Autodesk Inventor part; units mm, degrees
ref_plane "YZ Plane" through (0, 0, 0) normal (1, 0, 0) x (0, 1, 0)
ref_plane "XZ Plane" through (0, 0, 0) normal (0, 1, 0) x (-1, 0, 0)
ref_plane "XY Plane" through (0, 0, 0) normal (0, 0, 1) x (1, 0, 0)
sketch "Sketch1" plane through (0, 0, 0) normal (0, 1, 0) x (-1, 0, 0)
  arc A0 (0, -5) -> (4.4, -2.3749) centre (0, 0) ccw
  line L0 (0, 0) -> (0, 29.6022) construction
  line L1 (10, 9.2633) -> (10, 13.6302)
  line L2 (2.254, 28) -> (-1.8447, 28)
  line L3 (9.4, 6.8883) -> (4.4, -2.3749)
  arc A1 (9.4, 6.8883) -> (10, 9.2633) centre (5, 9.2633) ccw
  arc A2 (-4.4, -2.3749) -> (0, -5) centre (0, 0) ccw
  line L4 (-10, 9.2633) -> (-10, 23)
  line L5 (-5, 28) -> (-1.8447, 28)
  line L6 (-9.4, 6.8883) -> (-4.4, -2.3749)
  arc A3 (-10, 9.2633) -> (-9.4, 6.8883) centre (-5, 9.2633) ccw
  arc A4 (-5, 28) -> (-10, 23) centre (-5, 23) ccw
  arc A5 (4.825, 18) -> (6.95, 15.875) centre (6.95, 18) ccw
  line L7 (4.825, 18) -> (4.825, 28)
  line L8 (4.825, 28) -> (2.254, 28)
  line L9 (10, 13.6302) -> (10, 15.875)
  line L10 (10, 15.875) -> (6.95, 15.875)
  circle A6 centre (0, 0) radius 5
  point P0 (10, 28)
  point P1 (10, 8)
  point P2 (-10, 28)
  dimension "d0" = 10
  dimension "d3" = 10
  dimension "d4" = 28
  dimension "d26" = 8
  dimension "d27" = 5
  dimension "d48" = 5
  dimension "d51" = 3.05
  dimension "d52" = 10
  dimension "d53" = 4.25
extrude "Extrusion1" add sketch "Sketch1" along normal blind 2
sketch "Sketch3" plane through (0, 2, 0) normal (0, 1, 0) x (1, 0, 0)
  line L0 (0, 0) -> (0, -24.7147) construction
  line L1 (-4.825, -28) -> (5, -28)
  arc A0 (9.25, -8) -> (4.75, -8) centre (7, -8) ccw
  circle A1 centre (-7, -13.5) radius 2.25
  line L2 (7, -8) -> (7, -11) construction
  line L3 (9.25, -8) -> (9.25, -11)
  line L4 (4.75, -11) -> (4.75, -8)
  arc A2 (9.25, -8) -> (4.75, -8) centre (7, -8) ccw
  arc A3 (4.75, -11) -> (9.25, -11) centre (7, -11) ccw
  arc A4 (-6.5467, -11.2961) -> (5.1678, -6.694) centre (-4.2232, 0) ccw
  line L5 (7.3955, -13.215) -> (-6.6045, -15.715)
  point P0 (-4, -28)
  point P1 (-2.254, -28)
  point P2 (7, -9.5)
  dimension "d28" = 20
  dimension "d29" = 7
  dimension "d46" = 7
  dimension "d47" = 14.5
  dimension "d96" = 4.5
  dimension "d97" = 4.5
  dimension "d136" = 3
fillet "Fillet1" radius 2 2 edges at (-10, 1, 15.875) (-4.825, 1, 28)
sketch "Sketch4" plane through (0, 0, 0) normal (0, -1, 0) x (1, 0, 0)
  point P0 (0, 0)
  point P1 (0, 25)
  dimension "d37" = 25
hole "Hole4" at (0, 0, 25) direction (0, 1, 0) diameter 3 end through all
sketch "Sketch5" plane through (0, 0, 0) normal (0, -1, 0) x (1, 0, 0)
  circle A0 centre (0, 25) radius 1.5
  circle A1 centre (0, 25) radius 1.5
  arc A2 (-2.825, 28) -> (-4.825, 26) centre (-2.825, 26) ccw
  line L0 (-4.825, 26) -> (-4.825, 18)
  arc A3 (-6.95, 15.875) -> (-4.825, 18) centre (-6.95, 18) ccw
  line L1 (-6.95, 15.875) -> (-8, 15.875)
  arc A4 (-8, 15.875) -> (-10, 13.875) centre (-8, 13.875) ccw
  line L2 (-10, 13.875) -> (-10, 9.2633)
  arc A5 (-10, 9.2633) -> (-9.4, 6.8883) centre (-5, 9.2633) ccw
  line L3 (-9.4, 6.8883) -> (-4.4, -2.3749)
  arc A6 (-4.4, -2.3749) -> (4.4, -2.3749) centre (0, 0) ccw
  line L4 (4.4, -2.3749) -> (9.4, 6.8883)
  arc A7 (9.4, 6.8883) -> (10, 9.2633) centre (5, 9.2633) ccw
  line L5 (10, 9.2633) -> (10, 23)
  arc A8 (10, 23) -> (5, 28) centre (5, 23) ccw
  line L6 (5, 28) -> (-2.825, 28)
  circle A9 centre (0, 25) radius 9.8995 construction
  line L7 (0, 25) -> (17.632, 25) construction
  line L8 (0, 25) -> (13.9609, 10.961) construction
  arc A10 (4.6888, 20.285) -> (10, 16.7785) centre (6.9804, 17.9805) ccw
  arc A11 (4.6888, 20.285) -> (5.9826, 27.9025) centre (0, 25) ccw
  dimension "d55" = 19.799
  dimension "d56" = 45.16
  dimension "d57" = 6.5
extrude "Extrusion2" cut sketch "Sketch5" against normal through all contours A8 L5 A10 A11
fillet "Fillet2" radius 3 1 edges at (5.9826, 1, 27.9025)
fillet "Fillet3" radius 2 1 edges at (10, 1, 16.7785)
extrude "Extrusion5" add sketch "Sketch3" against normal blind 6.75
sketch "Sketch14" plane through (0, 0, 0) normal (0, -1, 0) x (1, 0, 0)
  circle A0 centre (0, 0) radius 5
  dimension "d123" = 10
extrude "Extrusion6" add sketch "Sketch14" along normal blind 1
sketch "Sketch15" plane through (0, -1, 0) normal (0, -1, 0) x (1, 0, 0)
  circle A0 centre (0, 0) radius 4.75
  dimension "d126" = 9.5
extrude "Extrusion7" add sketch "Sketch15" along normal blind 2.1
sketch "Sketch16" plane through (0, 2, 0) normal (0, 1, 0) x (1, 0, 0)
  point P0 (0, 0)
  point P1 (0, 0)
hole "Hole11" at (0, 2, 0) direction (0, -1, 0) diameter 3 end through all
sketch "Sketch17" plane through (0, -4.75, 0) normal (0, -1, 0) x (1, 0, 0)
  arc A0 (-6.6045, 15.715) -> (-6.5467, 11.2961) centre (-7, 13.5) ccw
  arc A1 (5.1678, 6.694) -> (-6.5467, 11.2961) centre (-4.2232, 0) ccw
  arc A2 (5.1678, 6.694) -> (9.25, 8) centre (7, 8) ccw
  line L0 (9.25, 8) -> (9.25, 11)
  arc A3 (9.25, 11) -> (7.3955, 13.215) centre (7, 11) ccw
  line L1 (7.3955, 13.215) -> (-6.6045, 15.715)
  line L2 (7, 8) -> (7, 11) construction
  point P0 (0, 0)
  point P1 (7, 9.5)
hole "mounting" at (7, -4.75, 9.5) at (-7, -4.75, 13.5) direction (0, 1, 0) diameter 2 depth 5.5
properties part number "phalanx_2_housing_R"
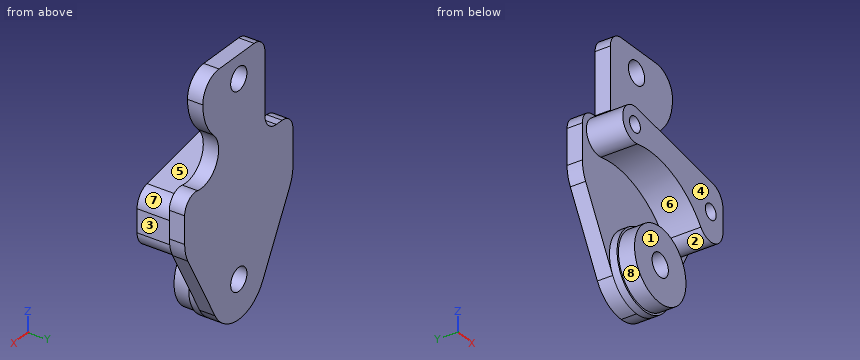
The model under review builds one solid part; all positions refer to its coordinate system, in mm. Face numbers are marked on the shaded views. A direction names the side the tool comes from. Give positions to 0.01 mm unless a question says otherwise; leave off trailing zeros. Order: outer loops, then holes, each group sorted by start corner. A loop starts at its lowest first (then second) coordinate and runs counter-clockwise, first axis right, second up. Notation, with made-up numbers: (-14, 32) - (32, 32) arc R22 ccw to (32, 70) - close; hole circle Ø4 at (73.5, 5). An arc over 180 degrees is marked (long way). Use CSV: the item, a comma, the result in double quotes. Start each with the question number.
Q1. The part is to be moulded in two halves that separate along X. For the marked faces 6, 7 and 8, say which applies: +X half, -X half, draft (parallel to the pull), parting line (faces both ways), or undercut.
Q2. We need section B-B, the plane x = 2.75. Write out the cut boundary in (y, z), and give its area (3 significant figures).
Q3. Tool access review of the marked faces 1, 2, 3, 4 and 5: name each direction out of +Z, -Z, +X, -X, +Y, -Y from which nothing blocks a thin tool from reaching the whole face with its end or side.
Q4. We need section C-C, the plane z = 2. Write out the cut boundary in (x, y).
Q5. We need section D-D, the plane x = 8.75. Write out the cut boundary in (y, z), and give its area (3 significant figures).
Q6. Clearance check with flat-ended pins moving along their axes: pin 1 Ø1 at (x, z) = (-1.5, 7.5) entering from -Y; pin 2 Ø10.5 at (x, z) = (0, 1) entering from -Y; pin 3 Ø1 at (y, z) = (1, 22) entering from -X (3 decimals). State where each tip first meets the part, or that it passes through.
Q7. To check wall thickness, follow line 1 along X through (y, z) = (1.15, 25) (3 decimals); line 2 along Z through (x, y) = (0, 0.9); line 3 along Y through (x, z) = (-8, 6.5). State the ranges of each line that lie inside material, in increasing order. Write a range as [from, to].
Q8. We need section A-A, the plane y = -2.25. State how many separate pieces and enclosed holes the cut face has, and give its area (3 significant figures).
Outcome:
1,face 6,"undercut"
1,face 7,"+X half"
1,face 8,"parting line"
2,outline,"(-4.75, 9.19) - (0, 9.19) - (0, 4.18) - (-1, 4.18) - (-1, 3.87) - (-3.1, 3.87) - (-3.1, -3.87) - (-1, -3.87) - (-1, -4.18) - (2, -4.18) - (2, 28) - (0, 28) - (0, 14.04) - (-4.75, 14.04) - close"
2,area,"112 mm^2"
3,face 1,"-Z, +X, -X, -Y"
3,face 2,"-Z, -Y"
3,face 3,"+Z, -Z, +X, -Y"
3,face 4,"+Z, -Z, +X, -X, -Y"
3,face 5,"+Z, +X, -Y"
4,outline,"(-6.76, 0) - (-4.58, 0) - (-4.58, -1) - (-4.31, -1) - (-4.31, -3.1) - (4.31, -3.1) - (4.31, -1) - (4.58, -1) - (4.58, 0) - (6.76, 0) - (6.76, 2) - (-6.76, 2) - close"
5,outline,"(-4.75, 6.59) - (0, 6.59) - (0, 5.68) - (2, 5.68) - (2, 14.68) - (0, 14.68) - (0, 12.41) - (-4.75, 12.41) - close"
5,area,"45.7 mm^2"
6,pin 1,"stops at y = 0"
6,pin 2,"stops at y = -3.1"
6,pin 3,"stops at x = -4.825"
7,line 1,"x = [-4.825, -1.5], [1.5, 6.65]"
7,line 2,"z = [-5, -1.5], [1.5, 23.5], [26.5, 28]"
7,line 3,"y = [0, 2]"
8,separate pieces,"2"
8,enclosed holes,"3"
8,area,"146 mm^2"
